Could you check a few things on this model? Use its own coordinates, in mm. A direction names the side the tool comes from. Coordinates: 2 decimals unless noted, no trailing zeros. Loops run counter-clockwise (first coordinate to the right, second up) from the corner with the lowest first, then second, coordinate; pieces in that order, holes last. Notation, with made-up numbers: M 23,-14 L 39,-14 A14 cw 39,11 Z; hole C 70.25,69.25 d8. An arc over 180 degrees is marked long. Use one line per item in the form item = value. Start each with the question number.
```python
from build123d import *

# Parameters (mm, degrees)
BOSS_EXTRUDE1_DEPTH             = 6.35
CUT_EXTRUDE1_REACH              = 46.798
SKETCH2_R                       = 3.175
BOSS_EXTRUDE2_REACH             = 46.798
SKETCH3_W                       = 15.648651434
SKETCH3_H                       = 6.35
BOSS_EXTRUDE2_DIRECTION_2_REACH = 46.798


with BuildPart() as part:
    # Sketch1 → Boss-Extrude1 (new body)
    with BuildSketch(Plane(origin=(0, 0, 0), x_dir=(1, 0, 0), z_dir=(0, 1, 0))):
        with BuildLine():
            Line((-25.172750094, -2.854782141), (-23.979365131, -3.554335257))
            Line((-23.979365131, -3.554335257), (-24.045420885, -4.814754144))
            Line((-24.045420885, -4.814754144), (-22.785001999, -4.880809899))
            Line((-22.785001999, -4.880809899), (-22.501080336, -6.110609729))
            Line((-22.501080336, -6.110609729), (-21.271280506, -5.826688067))
            Line((-21.271280506, -5.826688067), (-20.659378714, -6.930588121))
            Line((-20.659378714, -6.930588121), (-19.555478659, -6.318686329))
            Line((-19.555478659, -6.318686329), (-19.145844879, -7.284635532))
            Line((-19.145844879, -7.284635532), (-18.663004813, -6.38109418))
            Line((-18.663004813, -6.38109418), (-17.655008108, -7.140674179))
            Line((-17.655008108, -7.140674179), (-16.895428108, -6.132677474))
            Line((-16.895428108, -6.132677474), (-15.717110864, -6.584991086))
            Line((-15.717110864, -6.584991086), (-15.264797252, -5.406673842))
            Line((-15.264797252, -5.406673842), (-14.00745149, -5.516677342))
            Line((-14.00745149, -5.516677342), (-13.89744799, -4.259331581))
            Line((-13.89744799, -4.259331581), (-12.658488598, -4.018502271))
            Line((-12.658488598, -4.018502271), (-12.899317907, -2.779542878))
            Line((-12.899317907, -2.779542878), (-11.774735254, -2.206539397))
            Line((-11.774735254, -2.206539397), (-12.347738736, -1.081956744))
            Line((-12.347738736, -1.081956744), (-11.424661673, -0.221173456))
            Line((-11.424661673, -0.221173456), (-12.28544496, 0.701903607))
            Line((-12.28544496, 0.701903607), (-11.635390366, 1.783776131))
            Line((-11.635390366, 1.783776131), (-12.717262889, 2.433830725))
            Line((-12.717262889, 2.433830725), (-12.390594789, 3.652972671))
            Line((-12.390594789, 3.652972671), (-13.609736736, 3.979640771))
            Line((-13.609736736, 3.979640771), (-13.631764267, 5.241597158))
            Line((-13.631764267, 5.241597158), (-14.893720653, 5.219569627))
            Line((-14.893720653, 5.219569627), (-15.262737196, 6.426568353))
            Line((-15.262737196, 6.426568353), (-16.469735922, 6.05755181))
            Line((-16.469735922, 6.05755181), (-17.157151327, 7.116078708))
            Line((-17.157151327, 7.116078708), (-18.215678225, 6.428663303))
            Line((-18.215678225, 6.428663303), (-19.168233878, 7.256707299))
            Line((-19.168233878, 7.256707299), (-19.996277875, 6.304151646))
            Line((-19.996277875, 6.304151646), (-21.140172995, 6.837558701))
            Line((-21.140172995, 6.837558701), (-21.67358005, 5.69366358))
            Line((-21.67358005, 5.69366358), (-22.920189524, 5.891107124))
            Line((-22.920189524, 5.891107124), (-23.117633068, 4.64449765))
            Line((-23.117633068, 4.64449765), (-24.370373821, 4.490680427))
            Line((-24.370373821, 4.490680427), (-24.216556598, 3.237939674))
            Line((-24.216556598, 3.237939674), (-25.378370526, 2.412676209))
            Line((-25.378370526, 2.412676209), (-41.02702196, 2.557572596))
            Line((-41.02702196, 2.557572596), (-41.02702196, 10.177572596))
            Line((-41.02702196, 10.177572596), (-38.355583111, 10.177572596))
            ThreePointArc((-38.355583111, 10.177572596), (-33.547545085, 10.754594848), (-29.012572504, 12.452890476))
            Line((-29.012572504, 12.452890476), (-24.949455261, 14.556654192))
            ThreePointArc((-24.949455261, 14.556654192), (-18.492857296, 16.625923003), (-11.714907277, 16.455851756))
            Line((-11.714907277, 16.455851756), (33.40702196, 7.651462795))
            ThreePointArc((33.40702196, 7.651462795), (41.02702196, 0.031462795), (33.40702196, -7.588537205))
            Line((33.40702196, -7.588537205), (-12.038677684, -16.4558708))
            ThreePointArc((-12.038677684, -16.4558708), (-18.523682802, -16.66577615), (-24.744249109, -14.820808279))
            Line((-24.744249109, -14.820808279), (-29.229404705, -12.661591197))
            ThreePointArc((-29.229404705, -12.661591197), (-33.523201838, -11.159597642), (-38.043536354, -10.650427404))
            Line((-38.043536354, -10.650427404), (-41.02702196, -10.650427404))
            Line((-41.02702196, -10.650427404), (-41.02702196, -3.030427404))
            Line((-41.02702196, -3.030427404), (-25.172750094, -2.854782141))
        make_face()
    extrude(amount=BOSS_EXTRUDE1_DEPTH)

    # Sketch2 → Cut-Extrude1 (cut, up to next)
    with BuildSketch(Plane(origin=(0, 6.35, 0), x_dir=(1, 0, 0), z_dir=(0, 1, 0)), mode=Mode.PRIVATE) as cut_extrude1_sk1:
        with Locations(Location((33.40702196, 0.031462795, 0), (0, 0, 270))):
            Circle(SKETCH2_R)
    cut_extrude1_tool1 = extrude(cut_extrude1_sk1.sketch, amount=-CUT_EXTRUDE1_REACH, mode=Mode.PRIVATE) & part.part
    add(cut_extrude1_tool1.solids().sort_by_distance((33.407022, 6.35, -0.031463))[0], mode=Mode.SUBTRACT)

    # Sketch3 → Boss-Extrude2 (add, up to next)
    with BuildSketch(Plane.XY, mode=Mode.PRIVATE) as boss_extrude2_sk1:
        with Locations((-33.202696243, 3.175)):
            Rectangle(SKETCH3_W, SKETCH3_H)
    boss_extrude2_tool1 = extrude(boss_extrude2_sk1.sketch, amount=BOSS_EXTRUDE2_REACH, mode=Mode.PRIVATE) - part.part
    add(boss_extrude2_tool1.solids().sort_by_distance((-33.202696, 3.175, 0))[0])

    # Sketch3 → Boss-Extrude2 direction 2 (add, up to next)
    with BuildSketch(Plane.XY, mode=Mode.PRIVATE) as boss_extrude2_direction_2_sk1:
        with Locations((-33.202696243, 3.175)):
            Rectangle(SKETCH3_W, SKETCH3_H)
    boss_extrude2_direction_2_tool1 = extrude(boss_extrude2_direction_2_sk1.sketch, amount=-BOSS_EXTRUDE2_DIRECTION_2_REACH, mode=Mode.PRIVATE) - part.part
    add(boss_extrude2_direction_2_tool1.solids().sort_by_distance((-33.202696, 3.175, 0))[0])


solid = part.part
```
Item 1: For faces 5 (the flat face through (-40, 3, 10.65)), 6 (the flat face through (-40, 3, -10.178)), 7 (the flat face through (-1, 6.35, 0)), which set-ups out of +Z, -Z, +X, -X, +Y, -Y let a thin tool reach every point of the face, with its end or its side?
Item 2: I want a section at B-B (x = 0). Write out the boundary of the cut face in (y, z), plus the area to 3 significant figures.
Item 3: I want a section at C-C (x = -31). Write out the boundary of the cut face in (y, z), plus the area to 3 significant figures.
Item 4: I want a section at A-A (y = 2). Count the separate pieces of the cut face and the enclosed holes in it, plus the area to 3 significant figures.
Item 5: Please list where these lines run through material, in increasing order: line 1 along X through (y, z) = (3.75, 0); line 2 along X through (y, z) = (1.5, 1); line 3 along X through (y, z) = (2.75, -6.5).
Item 6: Thinking about a two-plate mould opening in Z: for faces 1 (the cylindrical face through (-33.61, 3.13, -10.74)), 2 (the flat face through (-26.955, 3.131, 13.756)), 3 (the flat face through (-1, 0, 0)), 4 (the flat face through (-25.378, 3, 0)), which applies, pulls with the +Z half, pulls with the -Z half, needs draft (parallel to the pull), parting line crosses it, or undercut?
Item 7: I'm going to push flat-ended pins straight in: P1, Ø1, axis at y = 5, z = -2.5, coming from the +X side; P2, Ø0.9, axis at x = -40, y = 2, coming from the +Z side; P3, Ø0.8, axis at x = -39.5, y = 2, coming from the -Z side. Where does each tip first touch, or does it pass through?
Worked answers:
q1.face_5 = +Z, -X, +Y, -Y
q1.face_6 = -Z, -X, +Y, -Y
q1.face_7 = +Z, -Z, +X, -X, +Y
q2.outline = M 0,-14.17 L 6.35,-14.17 L 6.35,14.11 L 0,14.11 Z
q2.area = 180 mm²
q3.outline = M 0,-11.56 L 6.35,-11.56 L 6.35,11.91 L 0,11.91 Z
q3.area = 149 mm²
q4.separate_pieces = 1
q4.enclosed_holes = 2
q4.area = 1,800 mm²
q5.line_1 = -41.03 to -25.38, -11.63 to 30.23, 36.58 to 41.03
q5.line_2 = -41.03 to -25.38, -12.26 to 30.4, 36.41 to 40.96
q5.line_3 = -41.03 to -21.3, -20.42 to -19.83, -18.3 to -18.11, -16.76 to 37.43
q6.face_1 = pulls with the -Z half
q6.face_2 = pulls with the +Z half
q6.face_3 = needs draft
q6.face_4 = undercut
q7.P1 = 40.77
q7.P2 = 10.65
q7.P3 = -10.18
